Here's how the part is built. I have some questions about the finished solid (model axes, mm). Face numbers are marked on the shaded views. A direction names the side the tool comes from. Round coordinates to 2 decimals unless told otherwise and drop trailing zeros. Loops run counter-clockwise (first coordinate to the right, second up) from the corner with the lowest first, then second, coordinate; pieces in that order, holes last. Notation, with made-up numbers: (-24, 15) - (-9, 15) arc R23 cw to (-9, 37) - close; hole circle Ø10 at (89, 45). An arc over 180 degrees is marked (long way). Answer as a JSON object with one key per item and string values. Group by question number.
1) I want a section at D-D, the plane y = 2.25. Please give me the cut outline in (x, z), then the cut area to 3 significant figures.
2) Will these pins go through, and if not, where does the flat tip stop? P1, Ø5, axis at y = 6, z = -32, coming from the -X side; P2, Ø7.5, axis at y = 7, z = -14, coming from the -X side; P3, Ø4, axis at y = 11, z = -30.5, coming from the -X side.
3) I want a section at C-C, the plane z = -9.5. Please give me the cut outline in (x, y).
4) Which directions (+Z, -Z, +X, -X, +Y, -Y) give clear straight access to the entire face, cutting with the end or side of a thin tool? Please do the marked faces 1 and 2.
5) I want a section at B-B, the plane y = 8.5. Please give me the cut outline in (x, z), then the cut area to 3 significant figures.
6) If I drill on line 1 along Y through (x, z) = (-2.65, -7.5); line 2 along X through (y, z) = (11, -48.5); line 3 along X through (y, z) = (11.75, -4.5), over which ranges is the centre line in solid material (lowest first)? Write a range as [from, to].
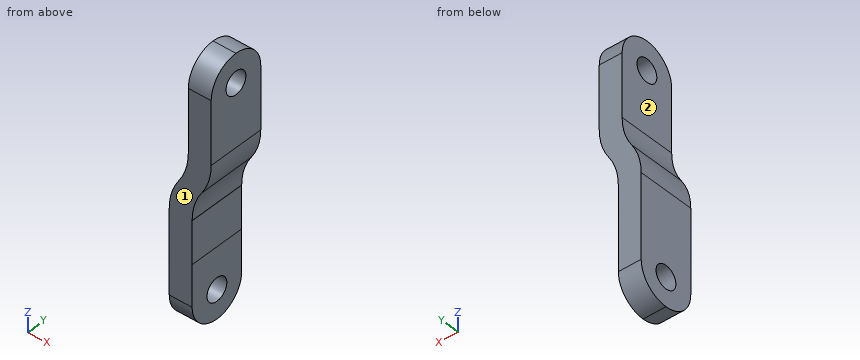
Autodesk Inventor part; units mm, degrees
ref_plane "YZ Plane" through (0, 0, 0) normal (1, 0, 0) x (0, 1, 0)
ref_plane "XZ Plane" through (0, 0, 0) normal (0, 1, 0) x (-1, 0, 0)
ref_plane "XY Plane" through (0, 0, 0) normal (0, 0, 1) x (1, 0, 0)
sketch "Sketch1" plane through (0, 0, 0) normal (0, 1, 0) x (-1, 0, 0)
  line L0 (0, 0) -> (6, 0)
  line L1 (6, 0) -> (76, 0) construction
  line L2 (6, -70) -> (5, -70)
  line L3 (5, -70) -> (5, -51.6792)
  line L4 (5, -70) -> (11, -70)
  line L5 (11, -70) -> (11, -40.5)
  line L6 (5.0002, -40.5) -> (5, -40.5)
  line L7 (5, -40.5) -> (5, -70)
  line L8 (6, 0) -> (6, -23.9152)
  line L9 (0, -23.9152) -> (0, 0)
  arc A0 (-0.0017, -54.956) -> (0, -54.9555) centre (-3.9998, -40.4987) ccw
  arc A1 (-0.0017, -51.6807) -> (0, -51.6792) centre (-9.9998, -40.4987) ccw
  arc A2 (5, -40.5731) -> (2.5001, -32.2069) centre (-9.9998, -40.4987) ccw
  arc A3 (11, -40.5731) -> (8.5001, -32.2069) centre (-3.9998, -40.4987) ccw
  arc A4 (6, -23.9152) -> (8.5001, -32.2069) centre (21, -23.9152) ccw
  arc A5 (0, -23.9152) -> (2.5001, -32.2069) centre (15, -23.9152) ccw
  point P0 (6, -29.3181)
  point P1 (0, -29.3181)
  dimension "d0" = 6
extrude "Extrusion1" add sketch "Sketch1" along normal blind 15 contours L0 L8 A4 A0 A5 L9 | A0 L5 L3 L7 A1 A5 | L5 L4 L2 L3 A0
fillet "Fillet1" radius 7.5 4 edges at (-3, 0, 0) (-3, 15, 0) (-5.5, 15, -70) (-5.5, 0, -70)
sketch "Sketch3" plane through (0, 0, -23.9152) normal (1, 0, 0) x (0, 0, -1)
  circle A0 centre (-16.4152, 7.5) radius 3
  arc A1 (-16.4152, 15) -> (-16.4152, 0) centre (-16.4152, 7.5) ccw
  line L0 (-16.4152, 15) -> (0, 15)
  circle A2 centre (38.5848, 7.5) radius 3
  arc A3 (38.5848, 0) -> (38.5848, 15) centre (38.5848, 7.5) ccw
  line L1 (16.6579, 15) -> (38.5848, 15)
  point P0 (-23.9152, 0)
  point P1 (-23.9152, 7.5)
  point P2 (46.0848, 7.5)
  dimension "d15" = 6
  dimension "d16" = 7.5
  dimension "d17" = 7.5
  dimension "d18" = 6
  dimension "d19" = 7.5
  dimension "d20" = 7.5
extrude "Extrusion2" cut sketch "Sketch3" against normal blind 15
properties part number "atividade_14A_uniao"
Outcome:
{
 "1": {"outline": "(-11, -67.86) - (-5, -67.86) - (-5, -51.68) - (-5, -40.5) arc R15 cw to (-2.5, -32.21) arc R15 ccw to (0, -23.92) - (0, -2.14) - (-6, -2.14) - (-6, -23.92) arc R15 cw to (-8.5, -32.21) arc R15 ccw to (-11, -40.5) - close", "area": "394 mm^2"},
 "2": {"P1": "x = -9.75", "P2": "x = -6", "P3": "x = -8.69"},
 "3": {"outline": "(-6, 0) - (0, 0) - (0, 5.26) - (-6, 5.26) - close; (-6, 9.74) - (0, 9.74) - (0, 15) - (-6, 15) - close"},
 "4": {"face 1": "+Z, -Z, +X, -X, -Y", "face 2": "+Z, -X, +Y, -Y"},
 "5": {"outline": "(-11, -69.93) - (-5, -69.93) - (-5, -65.33) - (-11, -65.33) - close; (-11, -59.67) - (-5, -59.67) - (-5, -51.68) - (-5, -40.5) arc R15 cw to (-2.5, -32.21) arc R15 ccw to (0, -23.92) - (0, -10.33) - (-6, -10.33) - (-6, -23.92) arc R15 cw to (-8.5, -32.21) arc R15 ccw to (-11, -40.5) - close; (-6, -4.67) - (0, -4.67) - (0, -0.07) - (-6, -0.07) - close", "area": "351 mm^2"},
 "6": {"line 1": "[0, 4.5], [10.5, 15]", "line 2": "[-11, -5]", "line 3": "[-6, 0]"}
}
